Here's how the part is built. I have some questions about the finished solid (model axes, mm). A direction names the side the tool comes from. Coordinates: 2 decimals unless noted, no trailing zeros. Order: outer loops, then holes, each group sorted by start corner. A loop starts at its lowest first (then second) coordinate and runs counter-clockwise, first axis right, second up. Notation, with made-up numbers: (88, 35) - (137, 35) arc R28 cw to (137, 55) - close; hole circle Ø1 at (67.25, 10.25). An arc over 180 degrees is marked (long way). Answer as CSV lines item,"result". Start each with the question number.
Q1. Suppose I cut it at C-C (x = -1). Please give me the cut outline in (y, z).
Q2. Suppose I cut it at B-B (z = 0). Please give me the cut outline in (x, y), then the cut area to 3 significant figures.
Q3. Suppose I cut it at A-A (y = -2.5). Please give me the cut outline in (x, z), then the cut area to 3 significant figures.
Q4. For pin 1 Ø10 at (y, z) = (-2.5, 5) entering from +X; pin 2 Ø4.5 at (x, y) = (-3, 7.5) entering from -Z; pin 3 Ø7.5 at (y, z) = (6.5, 1.5) entering from -X; pin 4 Ø1.5 at (x, z) = (0, 5) entering from +Y, each with a flat end and sliding along its axis, tell me the tip position at first contact or that it passes through.
Q5. Suppose I cut it at D-D (y = 6.25). Please give me the cut outline in (x, z).
Q6. I need wall thicknesses on line 1 (Z direction, x = 13, y = 0.25); line 2 (X direction, y = 0.25, z = 0.5); line 3 (Y direction, x = 7.5, z = 4.25). Which ranges of each line are inside material? Lowest first, please.
Q7. For faces 1 (the face through (-14, 7, 0)), 2 (the face through (-0.1, -3.1, 8.2)), 3 (the face through (0, 7, 4)), 4 (the face through (14, 7, 0)), which set-ups out of +Z, -Z, +X, -X, +Y, -Y let a thin tool reach every point of the face, with its end or its side?
from build123d import *

# Parameters (mm, degrees)
SKETCH_W     = 30
SKETCH_H     = 10
PAD_DEPTH    = 3.1
SKETCH001_W  = 40
SKETCH001_H  = 20
PAD001_DEPTH = 5
FILLET_R     = 1.5
FILLET001_R  = 3
FILLET002_R  = 1.5
SKETCH002_W  = 28
SKETCH002_H  = 8
PAD002_DEPTH = 14.9
FILLET003_R  = 0.5


with BuildPart() as part:
    # Sketch → Pad (new body)
    with BuildSketch(Plane.XZ):
        Rectangle(SKETCH_W, SKETCH_H)
    extrude(amount=PAD_DEPTH)

    # Sketch001 (on Face6 of Pad) → Pad001 (join)
    with BuildSketch(Plane.XZ.offset(3.1)):
        Rectangle(SKETCH001_W, SKETCH001_H)
    extrude(amount=PAD001_DEPTH)

    # Fillet
    fillet_edges = [part.edges().sort_by_distance(p)[0] for p in [
        (15, -1.55, 5),
        (15, -1.55, -5),
        (-15, -1.55, 5),
        (-15, -1.55, -5),
    ]]
    fillet(fillet_edges, radius=FILLET_R)

    # Fillet001
    fillet001_edges = [part.edges().sort_by_distance(p)[0] for p in [
        (0, -3.1, 5),
    ]]
    fillet(fillet001_edges, radius=FILLET001_R)

    # Fillet002
    fillet002_edges = [part.edges().sort_by_distance(p)[0] for p in [
        (0, -8.1, 10),
        (-20, -8.1, 0),
        (20, -8.1, 0),
        (0, -8.1, -10),
        (20, -5.6, 10),
        (-20, -5.6, 10),
        (20, -5.6, -10),
        (-20, -5.6, -10),
    ]]
    fillet(fillet002_edges, radius=FILLET002_R)

    # Sketch002 (on Face4 of Fillet001) → Pad002 (join)
    with BuildSketch(Plane(origin=(0, 0, 0), x_dir=(1, 0, 0), z_dir=(0, 1, 0))):
        Rectangle(SKETCH002_W, SKETCH002_H)
    extrude(amount=PAD002_DEPTH)

    # Fillet003
    fillet003_edges = [part.edges().sort_by_distance(p)[0] for p in [
        (14, 7.45, 4),
        (-14, 7.45, 4),
        (-14, 7.45, -4),
        (14, 7.45, -4),
    ]]
    fillet(fillet003_edges, radius=FILLET003_R)


solid = part.part
Here are the results:
1,outline,"(-8.1, -8.5) arc R1.5 ccw to (-6.6, -10) - (-3.1, -10) - (-3.1, -8) arc R3 cw to (-0.1, -5) - (0, -5) - (0, -4) - (14.9, -4) - (14.9, 4) - (0, 4) - (0, 5) - (-0.1, 5) arc R3 cw to (-3.1, 8) - (-3.1, 10) - (-6.6, 10) arc R1.5 ccw to (-8.1, 8.5) - close"
2,outline,"(-20, -6.6) arc R1.5 ccw to (-18.5, -8.1) - (18.5, -8.1) arc R1.5 ccw to (20, -6.6) - (20, -3.1) - (18, -3.1) arc R3 cw to (15, -0.1) - (15, 0) - (14, 0) - (14, 14.9) - (-14, 14.9) - (-14, 0) - (-15, 0) - (-15, -0.1) arc R3 cw to (-18, -3.1) - (-20, -3.1) - close"
2,area,"713 mm²"
3,outline,"(-16.2, -3.5) arc R2.7 ccw to (-13.5, -6.2) - (13.5, -6.2) arc R2.7 ccw to (16.2, -3.5) - (16.2, 3.5) arc R2.7 ccw to (13.5, 6.2) - (-13.5, 6.2) arc R2.7 ccw to (-16.2, 3.5) - close"
3,area,"396 mm²"
4,pin 1,"stops at x = 20"
4,pin 2,"stops at z = -4"
4,pin 3,"stops at x = -14"
4,pin 4,"stops at y = 0"
5,outline,"(-14, -3.5) arc R0.5 ccw to (-13.5, -4) - (13.5, -4) arc R0.5 ccw to (14, -3.5) - (14, 3.5) arc R0.5 ccw to (13.5, 4) - (-13.5, 4) arc R0.5 ccw to (-14, 3.5) - close"
6,line 1,"z = -4 to 4"
6,line 2,"x = -14 to 14"
6,line 3,"y = -8.1 to 0"
7,face 1,"+Z, -Z, -X, +Y"
7,face 2,"+Y"
7,face 3,"+Z, +X, -X, +Y"
7,face 4,"+Z, -Z, +X, +Y"
